The drawing under review shows one solid part. Ordinate dimensions are in mm from its lowest x, y, z. A direction names the side the tool comes from. Round coordinates to 2 decimals unless told otherwise and drop trailing zeros. Order: outer loops, then holes, each group sorted by start corner. A loop starts at its lowest first (then second) coordinate and runs counter-clockwise, first axis right, second up. Notation, with made-up numbers: M 84,-15.75 L 140,-15.75 A26 cw 140,0.25 Z; hole C 67.5,31.5 d5. An arc over 180 degrees is marked long. Answer as a JSON object with one key per item and string values. Group by question number.
1. To check wall thickness, follow probe 1 along Z at (x, y) = (7.75, 2.7); probe 2 along Y at (x, z) = (12.5, 2). State the ranges of each line that lie inside material, in increasing order. Write a range as [from, to].
2. Add section C-C on y = 1.9. State the section outline as (x, z) points, and give its area (3 significant figures).
3. Add section D-D on z = 4.75. State the section outline as (x, y) points.
4. Add section A-A on x = 11.75. State the section outline as (y, z) points.
5. Clearance check with flat-ended pins moving along their axes: P1, Ø0.8, axis at y = 1.5, z = 1, coming from the -X side; P2, Ø0.8, axis at x = 12, z = 19, coming from the +Y side; P3, Ø2, axis at x = 12, z = 1, coming from the -Y side. State where each tip first meets the part, or that it passes through.
6. Machinability: for the marked faces 1, 2, 3 and 4, which of the approach directions +Z, -Z, +X, -X, +Y, -Y give a long, thin tool a straight path to every point of the face, cutting with its end or side? Answer none if there is none.
7. Add section B-B on z = 6.75. State the section outline as (x, y) points.
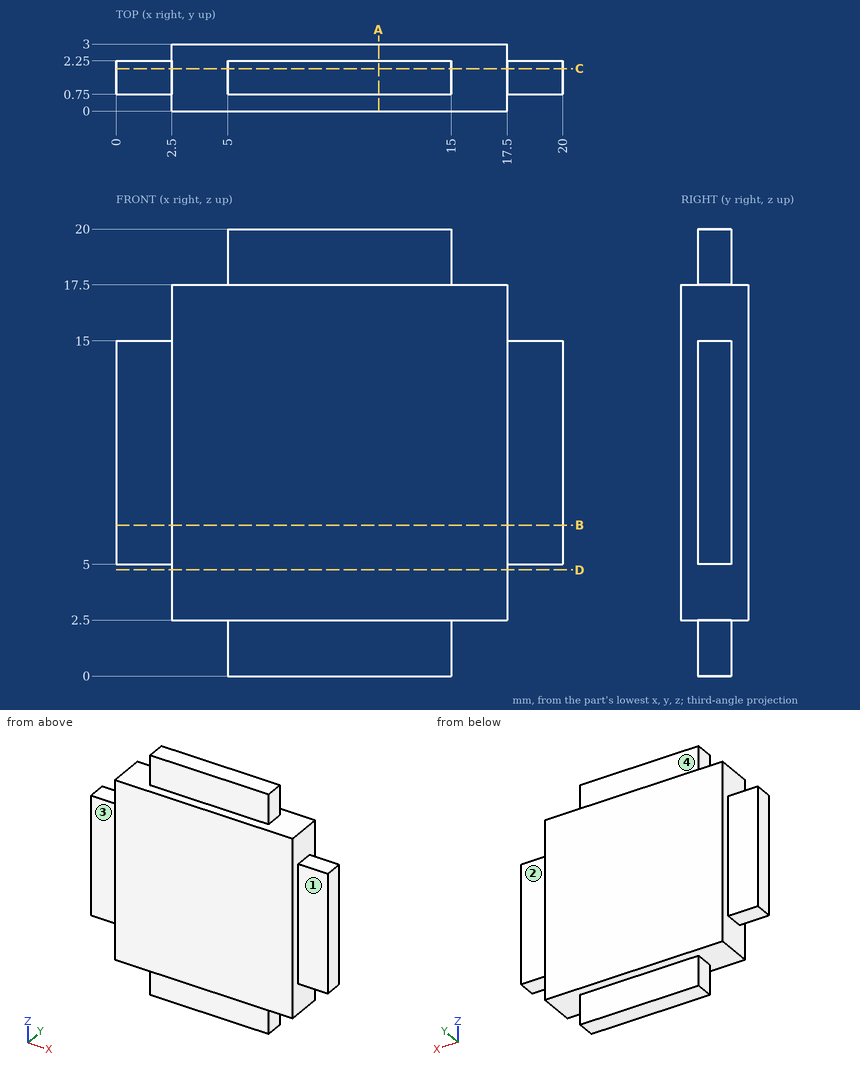
Recorded:
{
 "1": {"probe 1": "z = [2.5, 17.5]", "probe 2": "y = [0.75, 2.25]"},
 "2": {"outline": "M 0,5 L 2.5,5 L 2.5,2.5 L 5,2.5 L 5,0 L 15,0 L 15,2.5 L 17.5,2.5 L 17.5,5 L 20,5 L 20,15 L 17.5,15 L 17.5,17.5 L 15,17.5 L 15,20 L 5,20 L 5,17.5 L 2.5,17.5 L 2.5,15 L 0,15 Z", "area": "325 mm²"},
 "3": {"outline": "M 2.5,0 L 17.5,0 L 17.5,3 L 2.5,3 Z"},
 "4": {"outline": "M 0,2.5 L 0.75,2.5 L 0.75,0 L 2.25,0 L 2.25,2.5 L 3,2.5 L 3,17.5 L 2.25,17.5 L 2.25,20 L 0.75,20 L 0.75,17.5 L 0,17.5 Z"},
 "5": {"P1": "stops at x = 5", "P2": "stops at y = 2.25", "P3": "stops at y = 0.75"},
 "6": {"face 1": "+Z, -Z, +X, -Y", "face 2": "+Z, -Z, +X, +Y", "face 3": "+Z, -Z, -X, -Y", "face 4": "+Z, +X, -X, +Y"},
 "7": {"outline": "M 0,0.75 L 2.5,0.75 L 2.5,0 L 17.5,0 L 17.5,0.75 L 20,0.75 L 20,2.25 L 17.5,2.25 L 17.5,3 L 2.5,3 L 2.5,2.25 L 0,2.25 Z"}
}
